Model file for the job. Use its own axes, mm. Face numbers are marked on the shaded views. A direction names the side the tool comes from. Round coordinates to 2 decimals unless told otherwise and drop trailing zeros. Order: outer loops, then holes, each group sorted by start corner. A loop starts at its lowest first (then second) coordinate and runs counter-clockwise, first axis right, second up. Notation, with made-up numbers: (-35.75, 22.25) -> (9.25, 22.25) arc R21 cw to (9.25, 53.25) -> close; hole circle Ø11 at (21.25, 61). An arc over 180 degrees is marked (long way). Answer as CSV lines item,"result".
```python
from build123d import *

# Parameters (mm, degrees)
SKETCH1_R                = 16.9291
BOSS_EXTRUDE1_DEPTH      = 6.35
CUT_EXTRUDE1_DEPTH       = 25.769161343
CUT_EXTRUDE1_DEPTH_BACK  = 25.769161343
SKETCH2_R                = 0.809435985
BOSS_EXTRUDE3_DEPTH      = 77
BOSS_EXTRUDE3_DEPTH_BACK = 108
SKETCH3_R                = 4.7625


with BuildPart() as part:
    # Sketch1 → Boss-Extrude1 (new body)
    with BuildSketch(Plane(origin=(0, 0, 0), x_dir=(1, 0, 0), z_dir=(0, 1, 0))):
        with Locations(Location((0, 0, 0), (0, 0, 270))):
            Circle(SKETCH1_R)
    extrude(amount=BOSS_EXTRUDE1_DEPTH)

    # Sketch2 → Cut-Extrude1 (cut, two sides: drawn at the far end of the back side and taken through both)
    with BuildSketch(Plane.XY.offset(-CUT_EXTRUDE1_DEPTH_BACK)):
        Circle(SKETCH2_R)
    extrude(amount=CUT_EXTRUDE1_DEPTH + CUT_EXTRUDE1_DEPTH_BACK, mode=Mode.SUBTRACT)

    # Sketch3 → Boss-Extrude3 (add, two sides: drawn at the far end of the back side and taken through both)
    with BuildSketch(Plane(origin=(0, 6.35, 0), x_dir=(1, 0, 0), z_dir=(0, 1, 0)).offset(-BOSS_EXTRUDE3_DEPTH_BACK)):
        with Locations(Location((0, 0, 0), (0, 0, 270))):
            Circle(SKETCH3_R)
    extrude(amount=BOSS_EXTRUDE3_DEPTH + BOSS_EXTRUDE3_DEPTH_BACK)


solid = part.part
```
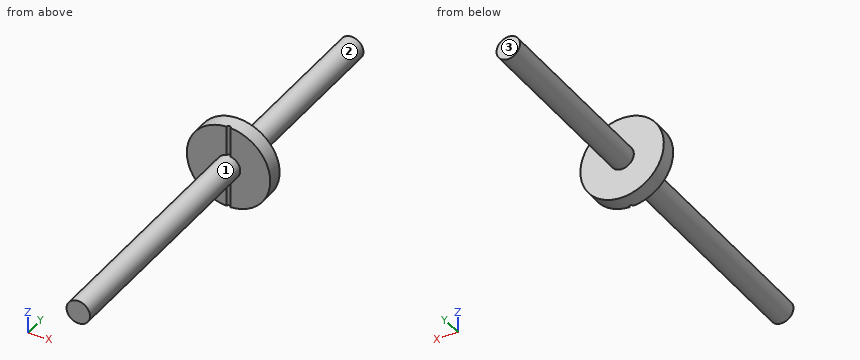
Q1. Saw through at D-D (z = 14.5). Write the cut outline in (x, y).
Checks:
outline,"(-8.74, 0) -> (-0.81, 0) arc R0.81 cw to (0.81, 0) -> (8.74, 0) -> (8.74, 6.35) -> (-8.74, 6.35) -> close"
Q2. Flat gauge pins, fed straight in: pin 1 (8 mm diameter, centred on x = 8, z = -5, fed in from -Y); pin 2 (8 mm diameter, centred on x = -3, z = 10.5, fed in from +Y); pin 3 (1.5 mm diameter, centred on x = -4.5, y = 5, fed in from -Z). Where does each tip first touch, or does it go through?
Checks:
pin 1,"y = 0"
pin 2,"y = 6.35"
pin 3,"z = -16.51"
Q3. Saw through at A-A (z = 0). Write the cut outline in (x, y), plus the area to 3 significant figures.
Checks:
outline,"(-16.93, 0) -> (-4.76, 0) -> (-4.76, -101.65) -> (4.76, -101.65) -> (4.76, 0) -> (16.93, 0) -> (16.93, 6.35) -> (4.76, 6.35) -> (4.76, 83.35) -> (-4.76, 83.35) -> (-4.76, 6.35) -> (-16.93, 6.35) -> close"
area,"1,920 mm²"
Q4. Tool access for the marked faces 1, 2 and 3: list every direction of +Z, -Z, +X, -X, +Y, -Y with a clear straight run to the whole face (end or side of a thin tool).
Checks:
face 1,"-Y"
face 2,"+Y"
face 3,"+Z, -Z, +X, -X, +Y"
Q5. Wall check: L1, parallel to Y at x = -10, z = 11; L2, parallel to Z at x = -1, y = 38.5; L3, parallel to X at y = -29.5, z = -4. Give the ranges that are in metal, low to high. Write a range as [from, to].
Checks:
L1,"[0, 6.35]"
L2,"[-4.66, 4.66]"
L3,"[-2.58, 2.58]"
Q6. Saw through at C-C (x = 10.5). Write the cut outline in (y, z).
Checks:
outline,"(0, -13.28) -> (6.35, -13.28) -> (6.35, 13.28) -> (0, 13.28) -> close"
Q7. Saw through at B-B (y = -10.5). Write the cut outline in (x, z) (1 decimal), plus the area to 3 significant figures.
Checks:
outline,"circle Ø9.5 at (0, 0)"
area,"71.3 mm²"
